```python
from build123d import *

# Parameters (mm, degrees)
EXTRUDE_1_DEPTH          = 22
FILLET_1_R               = 5
CHAMFER_1_SIZE           = 1
SKETCH_4_R               = 2.5
CUT_EXTRUDE_1_DEPTH      = 39.522720569
MIRROR_4_COPY_1_SKETCH_R = 2.5
MIRROR_4_COPY_1_DEPTH    = 39.522720569
CHAMFER_2_SIZE           = 0.5
HOLE_WIZARD_M5_1_D       = 4.2


with BuildPart() as part:
    # 草图1 → 凸台-拉伸1 (new, symmetric)
    with BuildSketch(Plane.XY):
        Polygon((-9, 0), (-30, 0), (-30, 8), (-16, 8), (-16, 18), (16, 18), (16, 8), (30, 8), (30, 0), (9, 0), (9, 11), (-9, 11), align=None)
    extrude(amount=EXTRUDE_1_DEPTH, both=True)

    # 圆角1
    fillet_1_edges = [part.edges().sort_by_distance(p)[0] for p in [
        (-30, 4, 22),
        (30, 4, 22),
        (30, 4, -22),
        (-30, 4, -22),
    ]]
    fillet(fillet_1_edges, radius=FILLET_1_R)

    # 倒角1
    chamfer_1_edges = [part.edges().sort_by_distance(p)[0] for p in [
        (-20.5, 8, 22),
        (0, 18, 22),
        (-16, 18, 0),
        (16, 18, 0),
        (0, 18, -22),
        (-30, 8, 0),
        (20.5, 8, -22),
        (-28.535533906, 8, 20.535533906),
        (-20.5, 8, -22),
        (-28.535533906, 8, -20.535533906),
        (30, 8, 0),
        (20.5, 8, 22),
        (28.535533906, 8, 20.535533906),
        (28.535533906, 8, -20.535533906),
    ]]
    chamfer(chamfer_1_edges, length=CHAMFER_1_SIZE)

    # 草图4 → 切除-拉伸1 (cut, through all)
    with BuildSketch(Plane(origin=(0, 8, 0), x_dir=(1, 0, 0), z_dir=(0, 1, 0))):
        with Locations(Location((22.5, 12.5, 0), (0, 0, 180))):
            Circle(SKETCH_4_R)
    cut_extrude_1 = extrude(amount=-CUT_EXTRUDE_1_DEPTH, mode=Mode.SUBTRACT)

    # 镜向3: 切除-拉伸1 across plane
    add(cut_extrude_1.mirror(Plane(origin=(0, 0, 0), x_dir=(0, 0, 1), z_dir=(1, 0, 0))), mode=Mode.SUBTRACT)

    # 镜向4: 切除-拉伸1 across plane
    add(cut_extrude_1.mirror(Plane.XY), mode=Mode.SUBTRACT)

    # 镜向4 copy 1 sketch → 镜向4 copy 1 (cut, through all)
    with BuildSketch(Plane(origin=(0, 8, 0), x_dir=(-1, 0, 0), z_dir=(0, 1, 0))):
        with Locations(Location((22.5, 12.5, 0), (0, 0, 180))):
            Circle(MIRROR_4_COPY_1_SKETCH_R)
    extrude(amount=-MIRROR_4_COPY_1_DEPTH, mode=Mode.SUBTRACT)

    # 倒角2
    chamfer_2_edges = [part.edges().sort_by_distance(p)[0] for p in [
        (25, 8, -12.5),
        (-25, 8, -12.5),
        (25, 8, 12.5),
        (-25, 8, 12.5),
    ]]
    chamfer(chamfer_2_edges, length=CHAMFER_2_SIZE)

    # M5 螺纹孔1 (through all)
    with Locations(Plane(origin=(0, 18, -9.540064206), x_dir=(1, 0, 0), z_dir=(0, 1, 0))):
        with Locations((0, 0)):
            hole_wizard_m5_1 = Hole(HOLE_WIZARD_M5_1_D / 2)

    # 镜向5: M5 螺纹孔1 across plane
    add(hole_wizard_m5_1.mirror(Plane.XY), mode=Mode.SUBTRACT)


solid = part.part
```
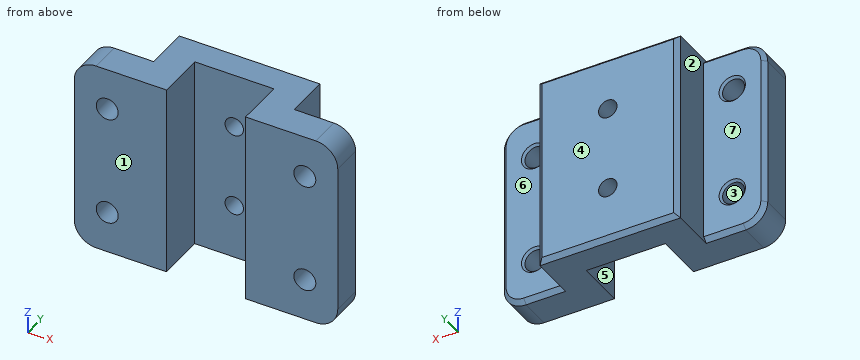
Source: CAD feature listing. Evaluate the final solid. Frame: model axes, mm. Face numbers are marked on the shaded views. A direction names the side the tool comes from. Coordinates: 2 decimals unless noted, no trailing zeros. Write each loop counter-clockwise with the first axis right and the second up, starting at its lowest first coordinate (ties: lowest second). Pieces come first, ordered by that corner, then holes. Notation, with made-up numbers: (41.5, 54.5) -> (96.5, 54.5) arc R19 ccw to (96.5, 60.5) -> close; hole circle Ø1 at (45, 28). An arc over 180 degrees is marked (long way). Return JSON: item names as keys, results as strings. Group by question number.
1) Section query B-B, the plane z = -12.5. Return loops of the section in (x, y), plus the area to 4 significant figures.
2) Contact query for flat-ended pins moving along their axis: P1, Ø4, axis at x = 24.5, z = -6, coming from the +Y side; P2, Ø14.5, axis at x = 0.5, z = -2, coming from the -Y side; P3, Ø4, axis at x = 22.5, z = 12.5, coming from the +Y side; P4, Ø4, axis at y = 12.5, z = -3, coming from the -X side. Output: stop coordinate, or through.
3) Mould query, pull axis X, two halves, no side actions, for the marked faces 1, 2 and 3. Classes: +X half, -X half, draft (parallel to the pull), parting line (faces both ways), or undercut.
4) Set-up query: the marked faces 4, 5, 6 and 7. Return all of +Z, -Z, +X, -X, +Y, -Y with unobstructed straight access to the full face (end or side cutting, diameter ignored); none if empty.
5) Section query C-C, the plane x = -22.5. Return loops of the section in (y, z).
6) Section query D-D, the plane y = 9.25. Return loops of the section in (x, z).
7) Ray query, line 1 along Z through (x, y) = (0, 13.5); line 2 along Z through (x, y) = (22.5, 1.5); line 3 along X through (y, z) = (4, 12.5). Return the intervals inside material, ascending.
8) Section query A-A, the plane y = 4.75. Return loops of the section in (x, z), plus the area to 3 significant figures.
From the geometry:
{
 "1": {"outline": "(-30, 0) -> (-25, 0) -> (-25, 7.5) -> (-25.5, 8) -> (-29, 8) -> (-30, 7) -> close; (-20, 0) -> (-9, 0) -> (-9, 11) -> (9, 11) -> (9, 0) -> (20, 0) -> (20, 7.5) -> (19.5, 8) -> (16, 8) -> (16, 17) -> (15, 18) -> (-15, 18) -> (-16, 17) -> (-16, 8) -> (-19.5, 8) -> (-20, 7.5) -> close; (25, 0) -> (30, 0) -> (30, 7) -> (29, 8) -> (25.5, 8) -> (25, 7.5) -> close", "area": "519.5 mm²"},
 "2": {"P1": "y = 8", "P2": "y = 11", "P3": "through", "P4": "x = -16"},
 "3": {"face 1": "draft", "face 2": "-X half", "face 3": "undercut"},
 "4": {"face 4": "+Z, -Z, +X, -X, +Y", "face 5": "+Z, -Z, -Y", "face 6": "+Z, -Z, +X, +Y", "face 7": "+Z, -Z, -X, +Y"},
 "5": {"outline": "(0, -22) -> (7, -22) -> (8, -21) -> (8, -15.5) -> (7.5, -15) -> (0, -15) -> close; (0, -10) -> (7.5, -10) -> (8, -9.5) -> (8, 9.5) -> (7.5, 10) -> (0, 10) -> close; (0, 15) -> (7.5, 15) -> (8, 15.5) -> (8, 21) -> (7, 22) -> (0, 22) -> close"},
 "6": {"outline": "(-16, -22) -> (-9, -22) -> (-9, 22) -> (-16, 22) -> close; (9, -22) -> (16, -22) -> (16, 22) -> (9, 22) -> close"},
 "7": {"line 1": "-22 to -11.64, -7.44 to 7.44, 11.64 to 22", "line 2": "-22 to -15, -10 to 10, 15 to 22", "line 3": "-30 to -25, -20 to -9, 9 to 20, 25 to 30"},
 "8": {"outline": "(-30, -17) arc R5 ccw to (-25, -22) -> (-9, -22) -> (-9, 22) -> (-25, 22) arc R5 ccw to (-30, 17) -> close; (9, -22) -> (25, -22) arc R5 ccw to (30, -17) -> (30, 17) arc R5 ccw to (25, 22) -> (9, 22) -> close; hole circle Ø5 at (-22.5, -12.5); hole circle Ø5 at (-22.5, 12.5); hole circle Ø5 at (22.5, -12.5); hole circle Ø5 at (22.5, 12.5)", "area": "1,750 mm²"}
}
